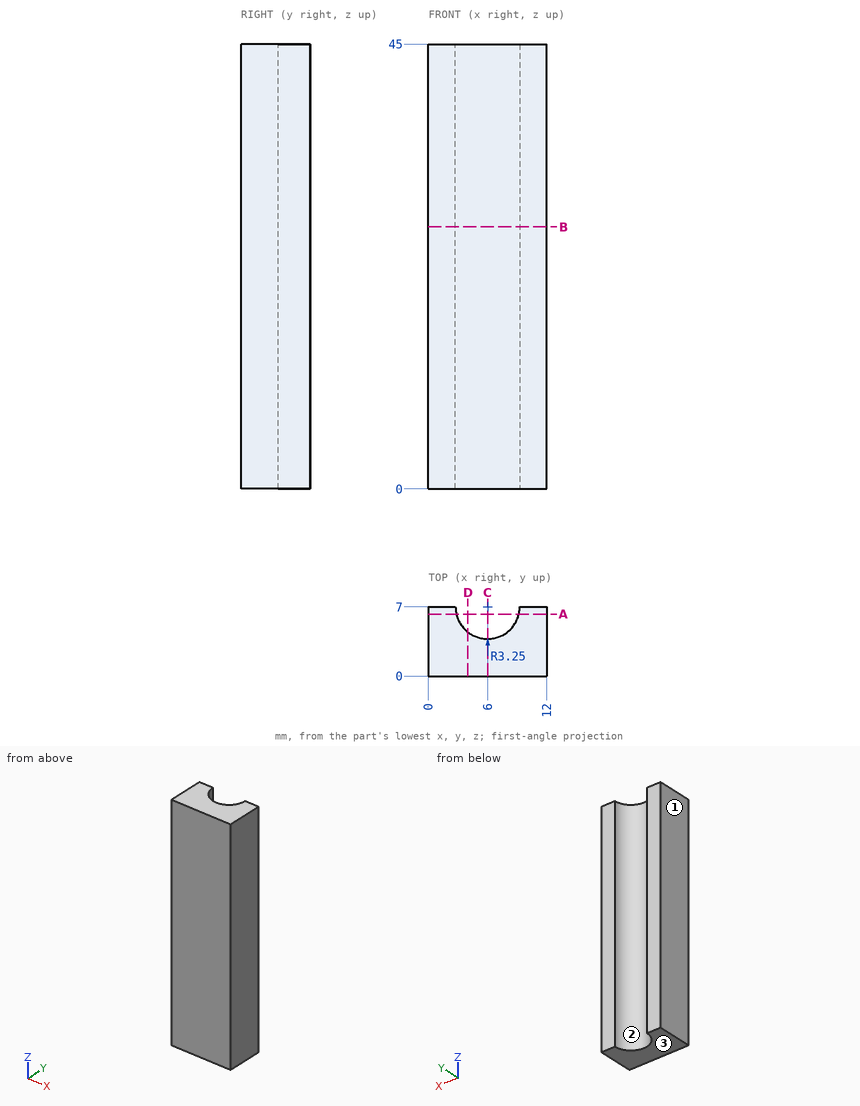
For this review, use the dimensioned drawing (mm, ordinates from the lowest corner) and the shaded views. Give positions to 0.01 mm unless a question says otherwise; leave off trailing zeros. Write each loop counter-clockwise with the first axis right and the second up, starting at its lowest first coordinate (ties: lowest second). Pieces come first, ordered by that corner, then holes. Notation, with made-up numbers: M 1,-34 L 7,-34 A10 ccw 7,-27 Z; hole C 3.25,-33.5 d9. An arc over 180 degrees is marked long. Answer as a JSON object with one key per item and string values. Group by question number.
Item 1: Consider section A-A on y = 6.25. Write out the cut boundary in (x, z).
Item 2: For pin 1 Ø1 at (x, z) = (10.5, 6) entering from -Y, flat-tipped, find the tip position at first contact; note if it passes through.
Item 3: For probe 1 along Y at (x, z) = (5.75, 20.5); probe 2 along X at (y, z) = (6, 5); probe 3 along X at (y, z) = (5.5, 31.5), list the stretches that pass through material, from the lowest coordinate up. Write a range as [from, to].
Item 4: Draft analysis for pull direction X (two halves, no side actions). For the marked faces 1, 2 and 3, state which applies: +X half, -X half, draft (parallel to the pull), parting line (faces both ways), or undercut.
Item 5: Consider section D-D on x = 4. Write out the cut boundary in (y, z), plus the area to 3 significant figures.
Item 6: Consider section B-B on z = 26.5. Write out the cut boundary in (x, y).
Item 7: Consider section C-C on x = 6. Write out the cut boundary in (y, z).
Check result:
{
 "1": {"outline": "M 0,0 L 2.84,0 L 2.84,45 L 0,45 Z; M 9.16,0 L 12,0 L 12,45 L 9.16,45 Z"},
 "2": {"pin 1": "stops at y = 0"},
 "3": {"probe 1": "y = [0, 3.76]", "probe 2": "x = [0, 2.91], [9.09, 12]", "probe 3": "x = [0, 3.12], [8.88, 12]"},
 "4": {"face 1": "-X half", "face 2": "undercut", "face 3": "draft"},
 "5": {"outline": "M 0,0 L 4.44,0 L 4.44,45 L 0,45 Z", "area": "200 mm^2"},
 "6": {"outline": "M 0,0 L 12,0 L 12,7 L 9.25,7 A3.25 cw 2.75,7 L 0,7 Z"},
 "7": {"outline": "M 0,0 L 3.75,0 L 3.75,45 L 0,45 Z"}
}
